Geometry check sheet. Reference: the model listing, model coordinates, mm. A direction names the side the tool comes from. Coordinates: 2 decimals unless noted, no trailing zeros. Loops run counter-clockwise (first coordinate to the right, second up) from the corner with the lowest first, then second, coordinate; pieces in that order, holes last.
from build123d import *

# Parameters (mm, degrees)
EXTRUDE_1_DEPTH     = 10
SKETCH_2_R          = 2
CUT_EXTRUDE_2_DEPTH = 10
CUT_EXTRUDE_3_DEPTH = 20


with BuildPart() as part:
    # 草图1 → 凸台-拉伸1 (new, symmetric)
    with BuildSketch(Plane.XY):
        with BuildLine():
            Line((0, 36), (0, 0))
            Line((0, 0), (28, 0))
            Line((28, 0), (28, 4.5))
            ThreePointArc((28, 4.5), (11.156427167, 16.552318383), (4.032383098, 36))
            Line((4.032383098, 36), (0, 36))
        make_face()
    extrude(amount=EXTRUDE_1_DEPTH, both=True)

    # 草图2 → 切除-拉伸2 (cut, symmetric)
    with BuildSketch(Plane(origin=(0, 0, 0), x_dir=(0, 0, -1), z_dir=(1, 0, 0))):
        with Locations((-5, 26)):
            Circle(SKETCH_2_R)
        with Locations((5, 26)):
            Circle(SKETCH_2_R)
    extrude(amount=CUT_EXTRUDE_2_DEPTH, both=True, mode=Mode.SUBTRACT)

    # 草图3 → 切除-拉伸3 (cut)
    with BuildSketch(Plane(origin=(5, 0, 0), x_dir=(0, 0, -1), z_dir=(1, 0, 0))):
        Polygon((-5, 30.041451884), (-8.5, 28.020725942), (-8.5, 23.979274058), (-5, 21.958548116), (-1.5, 23.979274058), (-1.5, 28.020725942), align=None)
        Polygon((5, 30.041451884), (1.5, 28.020725942), (1.5, 23.979274058), (5, 21.958548116), (8.5, 23.979274058), (8.5, 28.020725942), align=None)
    extrude(amount=CUT_EXTRUDE_3_DEPTH, mode=Mode.SUBTRACT)


solid = part.part
1) Mould release check, pull along Z, two halves, no side actions. Record for faces 3 (the cylindrical face through (2, 24, 5)), 4 (the flat face through (2, 36, 0)), 5 (the flat face through (8, 10, -10)): +Z half, -Z half, draft (parallel to the pull), parting line (faces both ways), or undercut.
Data:
face 3: undercut
face 4: draft
face 5: -Z half
2) Material ranges on probe 1 along Y at (x, z) = (2.7, -5); probe 2 along X at (y, z) = (28, -0.75); probe 3 along X at (y, z) = (26, 0.75), recorded low to high.
Data:
probe 1: y = 0 to 24, 28 to 36
probe 2: x = 0 to 5.39
probe 3: x = 0 to 6.03
3) Depth check by flat-ended pin: pin 1 (7.5 mm diameter, centred on y = 25.5, z = -5, fed in from +X); pin 2 (6 mm diameter, centred on x = 15.5, z = 2.5, fed in from +Y); pin 3 (8 mm diameter, centred on y = 23, z = 7.5, fed in from +X). Enter the tip coordinate at first touch or a pass-through.
Data:
pin 1: stops at x = 7.88
pin 2: stops at y = 14.89
pin 3: stops at x = 9.45
4) Access from +Z, -Z, +X, -X, +Y, -Y to the whole of each face (thin tool, end or side, straight path). Record for faces 1 (the flat face through (5.7, 25.6, 8.5)), 2 (the cylindrical face through (11.336, 16.319, 0.14)).
Data:
face 1: +X
face 2: +Z, -Z, +X, +Y
5) Section check D-D on y = 14. Record the cut outline in (x, z), and give its area (3 significant figures).
Data:
outline: (0, -10) - (13.3, -10) - (13.3, 10) - (0, 10) - close
area: 266 mm2
6) Section check C-C on x = 10. Record the cut outline in (y, z).
Data:
outline: (0, -10) - (18.16, -10) - (18.16, 10) - (0, 10) - close
7) Section check B-B on z = 0.25. Record the cut outline in (x, y).
Data:
outline: (0, 0) - (28, 0) - (28, 4.5) arc R35.12 cw to (4.03, 36) - (0, 36) - close
8) Section check A-A on y = 25. Record the cut outline in (x, z).
Data:
outline: (0, -10) - (6.41, -10) - (6.41, -8.5) - (5, -8.5) - (5, -6.73) - (0, -6.73) - close; (0, -3.27) - (5, -3.27) - (5, -1.5) - (6.41, -1.5) - (6.41, 1.5) - (5, 1.5) - (5, 3.27) - (0, 3.27) - close; (0, 6.73) - (5, 6.73) - (5, 8.5) - (6.41, 8.5) - (6.41, 10) - (0, 10) - close
